Could you check a few things on this model? Use its own coordinates, in mm. A direction names the side the tool comes from. Give positions to 0.01 mm unless a question says otherwise; leave off trailing zeros. Loops run counter-clockwise (first coordinate to the right, second up) from the corner with the lowest first, then second, coordinate; pieces in that order, holes last. Notation, with made-up numbers: M 62.25,47 L 110.25,47 A22 cw 110.25,82 Z; hole C 34.5,7.25 d4. An arc over 180 degrees is marked long. Answer in a Markdown table with one row per item. Add a question column.
1. I'm going to push flat-ended pins straight in: pin 1 Ø1.5 at (y, z) = (44, 15) entering from +X; pin 2 Ø14.5 at (x, z) = (-47.752, 0) entering from -Y; pin 3 Ø6 at (y, z) = (43.5, -4) entering from +X; pin 4 Ø4 at (x, y) = (-15, 24.5) entering from +Z. Where does each tip first touch, or does it pass through?
2. Which directions (+Z, -Z, +X, -X, +Y, -Y) give clear straight access to the entire face, cutting with the end or side of a thin tool? Please do faces 1 (the cylindrical face through (24.834, 34.542, -5.333)), 2 (the cylindrical face through (-24.664, 38.606, -6.072)), 3 (the flat face through (0, 0, -15)), 4 (the cylindrical face through (-63.5, 13.4, -0.2)), 5 (the cylindrical face through (-25.4, 3.1, -0.1)).
3. If we section it at B-B on x = -52: List the corners of the cut face in (y, z) for me, then the cut area to 3 significant figures.
4. I need wall thicknesses on line 1 along Y through (x, z) = (29, -20); line 2 along X through (y, z) = (32, -11). Which ranges of each line are inside material? Lowest first, please. Write a range as from..to.
5. If we section it at C-C on z = 12: List the corners of the cut face in (x, y) for me, then the cut area to 3 significant figures.
6. If we section it at A-A on z = 3.5: List the corners of the cut face in (x, y) for me.
7. If we section it at D-D on y = 38: List the corners of the cut face in (x, z) for me, then the cut area to 3 significant figures.
8. Thinking about a two-plate mould opening in X: for faces 6 (the cylindrical face through (1.858, 28.175, -14.153)), 7 (the cylindrical face through (25.39, 3.13, 0.64)), 8 (the cylindrical face through (-41.41, 13.36, -0.28)), 9 (the flat face through (37, 6.35, 0)), which applies, released by +X, released by -X, zero draft, split by the parting line, or undercut?
```python
from build123d import *

# Parameters (mm, degrees)
SKETCH3_W                  = 118.872
SKETCH3_H                  = 41.148
CUT_EXTRUDE1_DEPTH         = 107.4453968
SKETCH4_W                  = 119.061805732
SKETCH4_H                  = 41.402
CUT_EXTRUDE2_DEPTH         = 107.4453968
F_1_2_1_124_DOWEL_HOLE1_D  = 28.5496
F_1_2_0_5000_DOWEL_HOLE1_D = 12.7
CHAMFER1_SIZE              = 22.352


with BuildPart() as part:
    # Sketch2 → Revolve1 (revolve)
    with BuildSketch(Plane.XY, mode=Mode.PRIVATE) as revolve1_sk:
        Polygon((-63.5, 20.574), (-63.5, 6.35), (-25.4, 6.35), (-25.4, 0), (0, 0), (0, 57.15), (-25.4, 57.15), (-25.4, 20.574), align=None)
    revolve(revolve1_sk.sketch.rotate(Axis((0, 0, 0), (0, 1, 0)), 180), axis=Axis((0, 0, 0), (0, 1, 0)))

    # Sketch3 → Cut-Extrude1 (cut, through all)
    with BuildSketch(Plane(origin=(0, 57.15, 0), x_dir=(1, 0, 0), z_dir=(0, 1, 0))):
        with Locations((0, -42.926)):
            Rectangle(SKETCH3_W, SKETCH3_H)
    extrude(amount=-CUT_EXTRUDE1_DEPTH, mode=Mode.SUBTRACT)

    # Sketch4 → Cut-Extrude2 (cut, through all)
    with BuildSketch(Plane(origin=(0, 57.15, 0), x_dir=(1, 0, 0), z_dir=(0, 1, 0))):
        with Locations((0, 42.799)):
            Rectangle(SKETCH4_W, SKETCH4_H)
    extrude(amount=-CUT_EXTRUDE2_DEPTH, mode=Mode.SUBTRACT)

    # 1/2 (1.124) Dowel Hole1 (through all)
    with Locations(Plane(origin=(0, 57.15, 0), x_dir=(1, 0, 0), z_dir=(0, 1, 0))):
        with Locations((0, 0)):
            Hole(F_1_2_1_124_DOWEL_HOLE1_D / 2)

    # 1/2 (0.5000) Dowel Hole1 (through all)
    with Locations(Plane(origin=(0, 20.574, 0), x_dir=(1, 0, 0), z_dir=(0, 1, 0))):
        with Locations((-47.752, 0), (47.752, 0)):
            Hole(F_1_2_0_5000_DOWEL_HOLE1_D / 2)

    # Chamfer1
    # the kernel refuses this chamfer: 22.352 mm, written as the material it takes off along each edge
    with BuildSketch(Plane(origin=(-69.546589707, 57.15, 22.352), x_dir=(0, -0.9996219169112968, 0.027495876610586365), z_dir=(1, 0, 0))) as chamfer1_piece_1:
        Polygon((CHAMFER1_SIZE * 0.999621916911, CHAMFER1_SIZE * 0.0274958766106), (-CHAMFER1_SIZE * 0.0274958766106, CHAMFER1_SIZE * 0.999621916911), (0, 0), align=None)
    extrude(amount=139.093179415, mode=Mode.SUBTRACT)


solid = part.part
```
Results:
| question | item | result |
|---|---|---|
| 1 | pin 1 | through |
| 1 | pin 2 | y = 6.35 |
| 1 | pin 3 | x = 25.38 |
| 1 | pin 4 | z = 21.82 |
| 2 | face 1 | +X, +Y |
| 2 | face 2 | -X, +Y |
| 2 | face 3 | +Z, -Z, +X, -X, -Y |
| 2 | face 4 | -X, +Y, -Y |
| 2 | face 5 | -X, -Y |
| 3 | outline | M 6.35,-22.1 L 20.57,-22.1 L 20.57,-4.72 L 6.35,-4.72 Z; M 6.35,4.72 L 20.57,4.72 L 20.57,22.35 L 6.35,22.35 Z |
| 3 | area | 498 mm2 |
| 4 | line 1 | 6.35..20.57 |
| 4 | line 2 | -22.89..-9.1, 9.1..22.89 |
| 5 | outline | M -62.36,6.35 L -22.39,6.35 L -22.39,0 L -7.73,0 L -7.73,45.15 L -22.39,45.15 L -22.39,20.57 L -62.36,20.57 Z; M 7.73,0 L 22.39,0 L 22.39,6.35 L 62.36,6.35 L 62.36,20.57 L 22.39,20.57 L 22.39,45.15 L 7.73,45.15 Z |
| 5 | area | 2,460 mm2 |
| 6 | outline | M -63.4,6.35 L -53.05,6.35 L -53.05,20.57 L -63.4,20.57 Z; M -42.45,6.35 L -25.16,6.35 L -25.16,0 L -13.84,0 L -13.84,53.65 L -25.16,53.65 L -25.16,20.57 L -42.45,20.57 Z; M 13.84,0 L 25.16,0 L 25.16,6.35 L 42.45,6.35 L 42.45,20.57 L 25.16,20.57 L 25.16,53.65 L 13.84,53.65 Z; M 53.05,6.35 L 63.4,6.35 L 63.4,20.57 L 53.05,20.57 Z |
| 7 | outline | M -16.69,19.15 A25.4 ccw -12.52,-22.1 L 12.52,-22.1 A25.4 ccw 16.69,19.15 Z; hole C 0,0 d28.55 |
| 7 | area | 1,190 mm2 |
| 8 | face 6 | undercut |
| 8 | face 7 | released by +X |
| 8 | face 8 | undercut |
| 8 | face 9 | zero draft |
